from build123d import *

# Parameters (mm, degrees)
SKETCH1_R           = 1.7145
BOSS_EXTRUDE1_DEPTH = 3.175


with BuildPart() as part:
    # Sketch1 → Boss-Extrude1 (new body)
    with BuildSketch(Plane(origin=(0, 0, 0), x_dir=(1, 0, 0), z_dir=(0, 1, 0))):
        Polygon((-38.1, 0), (-38.1, 23.6855), (-34.925, 23.6855), (-34.925, 21.463), (-32.385, 21.463), (-32.385, 23.6855), (-27.305, 23.6855), (-27.305, 27.1145), (-32.385, 27.1145), (-32.385, 29.337), (-34.925, 29.337), (-34.925, 27.1145), (-38.1, 27.1145), (-38.1, 38.1), (-41.275, 38.1), (-41.275, 63.5), (-38.1, 63.5), (-38.1, 74.4855), (-34.925, 74.4855), (-34.925, 72.263), (-32.385, 72.263), (-32.385, 74.4855), (-27.305, 74.4855), (-27.305, 77.9145), (-32.385, 77.9145), (-32.385, 80.137), (-34.925, 80.137), (-34.925, 77.9145), (-38.1, 77.9145), (-38.1, 88.9), (-12.7, 88.9), (-12.7, 92.075), (12.7, 92.075), (12.7, 88.9), (38.1, 88.9), (38.1, 77.9145), (34.925, 77.9145), (34.925, 80.137), (32.385, 80.137), (32.385, 77.9145), (27.305, 77.9145), (27.305, 74.4855), (32.385, 74.4855), (32.385, 72.263), (34.925, 72.263), (34.925, 74.4855), (38.1, 74.4855), (38.1, 63.5), (41.275, 63.5), (41.275, 38.1), (38.1, 38.1), (38.1, 27.1145), (34.925, 27.1145), (34.925, 29.337), (32.385, 29.337), (32.385, 27.1145), (27.305, 27.1145), (27.305, 23.6855), (32.385, 23.6855), (32.385, 21.463), (34.925, 21.463), (34.925, 23.6855), (38.1, 23.6855), (38.1, 0), align=None)
        with Locations(Location((-38.735, 50.8, 0), (0, 0, 270))):
            Circle(SKETCH1_R, mode=Mode.SUBTRACT)
        with Locations(Location((0, 89.535, 0), (0, 0, 270))):
            Circle(SKETCH1_R, mode=Mode.SUBTRACT)
        with Locations(Location((38.735, 50.8, 0), (0, 0, 270))):
            Circle(SKETCH1_R, mode=Mode.SUBTRACT)
    extrude(amount=BOSS_EXTRUDE1_DEPTH)


solid = part.part
Check sheet for the modelled part. Datum: model origin and axes. Units: mm. A direction names the side the tool comes from. Give positions to 0.01 mm unless a question says otherwise; leave off trailing zeros. Write each loop counter-clockwise with the first axis right and the second up, starting at its lowest first coordinate (ties: lowest second). Pieces come first, ordered by that corner, then holes. Notation, with made-up numbers: (21, -6.5) -> (27, -6.5) arc R24 cw to (27, 22.5) -> close; hole circle Ø1 at (31, 32). An arc over 180 degrees is marked (long way). One line per item, written item: value. Start each with the question number.
Item 1: Gauge pin test, flat ends, axial feed: pin 1 (1.6 mm diameter, centred on x = 37, y = 1.5, fed in from +Z); pin 2 (1.6 mm diameter, centred on y = 1, z = -10.5, fed in from +X); pin 3 (1 mm diameter, centred on y = 1.5, z = -25, fed in from +X) (3 decimals); pin 4 (1.6 mm diameter, centred on x = -29.5, y = 2, fed in from -Z). Record the tip position at first contact, or that the pin passes through.
Item 2: Section check D-D on y = 0.65. State how many separate pieces and enclosed holes the cut face has, then the cut area to 3 significant figures.
Item 3: Section check A-A on z = -50.8. Record the cut outline in (x, y) (1 decimal).
Item 4: Section check C-C on z = -86. Record the cut outline in (x, y) (3 decimals).
Item 5: Material ranges on probe 1 along Z at (x, y) = (-36.5, 1.3); probe 2 along X at (y, z) = (2.05, -50.8) (1 decimal); probe 3 along X at (y, z) = (2.4, -64), recorded low to high. Write a range as from..to.
Item 6: Section check B-B on x = 0. Record the cut outline in (y, z) (1 decimal).
Item 7: Tool access check on faces 4 (the flat face through (-32.385, 2, -23)), 5 (the flat face through (-27.305, 2, -25)), 6 (the flat face through (27.305, 2, -76)), 7 (the flat face through (-38.1, 2, -83)). Record the directions out of +Z, -Z, +X, -X, +Y, -Y that give a thin tool (end or side, any length) a straight path to the whole face; none if there is none.
Item 8: Draft check along Z on faces 1 (the flat face through (37, 2, -77.914)), 2 (the flat face through (-38.1, 2, -69)), 3 (the flat face through (25, 2, -88.9)). Enter one of: +Z half, -Z half, draft (parallel to the pull), parting line (faces both ways), or undercut.
Results list:
1. pin 1: z = 0
1. pin 2: x = 38.1
1. pin 3: x = 27.305
1. pin 4: z = -88.9
2. separate pieces: 1
2. enclosed holes: 3
2. area: 6,800 mm²
3. outline: (-41.3, 0) -> (-40.4, 0) -> (-40.4, 3.2) -> (-41.3, 3.2) -> close; (-37, 0) -> (37, 0) -> (37, 3.2) -> (-37, 3.2) -> close; (40.4, 0) -> (41.3, 0) -> (41.3, 3.2) -> (40.4, 3.2) -> close
4. outline: (-38.1, 0) -> (38.1, 0) -> (38.1, 3.175) -> (-38.1, 3.175) -> close
5. probe 1: -88.9..-77.91, -74.49..-27.11, -23.69..0
5. probe 2: -41.3..-40.4, -37..37, 40.4..41.3
5. probe 3: -38.1..38.1
6. outline: (0, -92.1) -> (3.2, -92.1) -> (3.2, -91.2) -> (0, -91.2) -> close; (0, -87.8) -> (3.2, -87.8) -> (3.2, 0) -> (0, 0) -> close
7. face 4: +Y, -Y
7. face 5: -X, +Y, -Y
7. face 6: +X, +Y, -Y
7. face 7: -Z, -X, +Y, -Y
8. face 1: undercut
8. face 2: draft
8. face 3: -Z half
